Geometry: final body of the model. Coordinates: model frame, mm. Give positions to 0.01 mm unless a question says otherwise; leave off trailing zeros. Order: outer loops, then holes, each group sorted by start corner. A loop starts at its lowest first (then second) coordinate and runs counter-clockwise, first axis right, second up. Notation, with made-up numbers: (4, 54) -> (23, 54) arc R27 ccw to (23, 75) -> close; hole circle Ø6 at (38, 48.5). An arc over 180 degrees is marked (long way). Write item = value, one per line.
Autodesk Inventor part; units mm, degrees
ref_plane "YZ Plane" through (0, 0, 0) normal (1, 0, 0) x (0, 1, 0)
ref_plane "XZ Plane" through (0, 0, 0) normal (0, 1, 0) x (-1, 0, 0)
ref_plane "XY Plane" through (0, 0, 0) normal (0, 0, 1) x (1, 0, 0)
sketch "Sketch1" plane through (0, 0, 0) normal (0, 1, 0) x (-1, 0, 0)
  circle A0 centre (0, 0) radius 9.525
  circle A1 centre (0, 0) radius 3.175
  circle A2 centre (4.7625, 4.7625) radius 1.5875
  circle A3 centre (-4.7625, 4.7625) radius 1.5875
  circle A4 centre (-4.7625, -4.7625) radius 1.5875
  circle A5 centre (4.7625, -4.7625) radius 1.5875
  dimension "d0" = 19.05
  dimension "d1" = 6.35
  dimension "d2" = 3.175
  dimension "d5" = 360
extrude "Extrusion1" add sketch "Sketch1" along normal blind 5.08
properties part number "Contracting Finger Motion Ring (motor to shaft)"
1) Section query C-C (x = -6). Output: boundary loops of the cut face in (y, z), plus the area to 3 significant figures.
Check sheet entries:
outline = (0, -7.4) -> (5.08, -7.4) -> (5.08, -5.76) -> (0, -5.76) -> close; (0, -3.77) -> (5.08, -3.77) -> (5.08, 3.77) -> (0, 3.77) -> close; (0, 5.76) -> (5.08, 5.76) -> (5.08, 7.4) -> (0, 7.4) -> close
area = 55.0 mm²
2) Section query D-D (y = 0.55). Count the separate pieces of the cut face and the enclosed holes in it, plus the area to 3 significant figures.
Check sheet entries:
separate_pieces = 1
enclosed_holes = 5
area = 222 mm²
3) Mould query, pull axis Z, two halves, no side actions, for faces 1 (the face through (4.969, 2.504, -6.336)), 2 (the face through (7.559, 2.504, 5.796)), 3 (the face through (-5.62, 2.5, -6.1)), 4 (the face through (-4, 5.08, 0)). Classes: +Z half, -Z half, draft (parallel to the pull), parting line (faces both ways), or undercut.
Check sheet entries:
face_1 = undercut
face_2 = parting line
face_3 = undercut
face_4 = draft
4) Section query A-A (x = 0). Output: boundary loops of the cut face in (y, z) (3 decimals).
Check sheet entries:
outline = (0, -9.525) -> (5.08, -9.525) -> (5.08, -3.175) -> (0, -3.175) -> close; (0, 3.175) -> (5.08, 3.175) -> (5.08, 9.525) -> (0, 9.525) -> close
5) Section query B-B (z = 0). Output: boundary loops of the cut face in (x, y) (3 decimals), plus the area to 3 significant figures.
Check sheet entries:
outline = (-9.525, 0) -> (-3.175, 0) -> (-3.175, 5.08) -> (-9.525, 5.08) -> close; (3.175, 0) -> (9.525, 0) -> (9.525, 5.08) -> (3.175, 5.08) -> close
area = 64.5 mm²
6) Line query: line 1 (X direction, y = 3.3, z = -4); line 2 (Z direction, x = -3.5, y = 1.3). Output: solid intervals per line, ascending. Write a range as from..to.
Check sheet entries:
line_1 = -8.64..-6.15, -3.37..3.37, 6.15..8.64
line_2 = -8.86..-5.72, -3.8..3.8, 5.72..8.86
7) First-contact query: P1, Ø2, axis at x = 3.5, y = 3.5, coming from the -Z side; P2, Ø4, axis at x = -4.76, z = 4.76, coming from the +Y side; P3, Ø3, axis at x = 3, y = 3.5, coming from the -Z side; P4, Ø1, axis at x = -1, y = 2, coming from the -Z side. Flat tips, straight axial feed; report the tip coordinate or a pass-through.
Check sheet entries:
P1 = -9.19
P2 = 5.08
P3 = -9.41
P4 = -9.51
